Could you check a few things on this drawing? It's one solid part, dimensions in mm from its lowest x, y, z. A direction names the side the tool comes from. Give positions to 0.01 mm unless a question says otherwise; leave off trailing zeros. Order: outer loops, then holes, each group sorted by start corner. A loop starts at its lowest first (then second) coordinate and runs counter-clockwise, first axis right, second up.
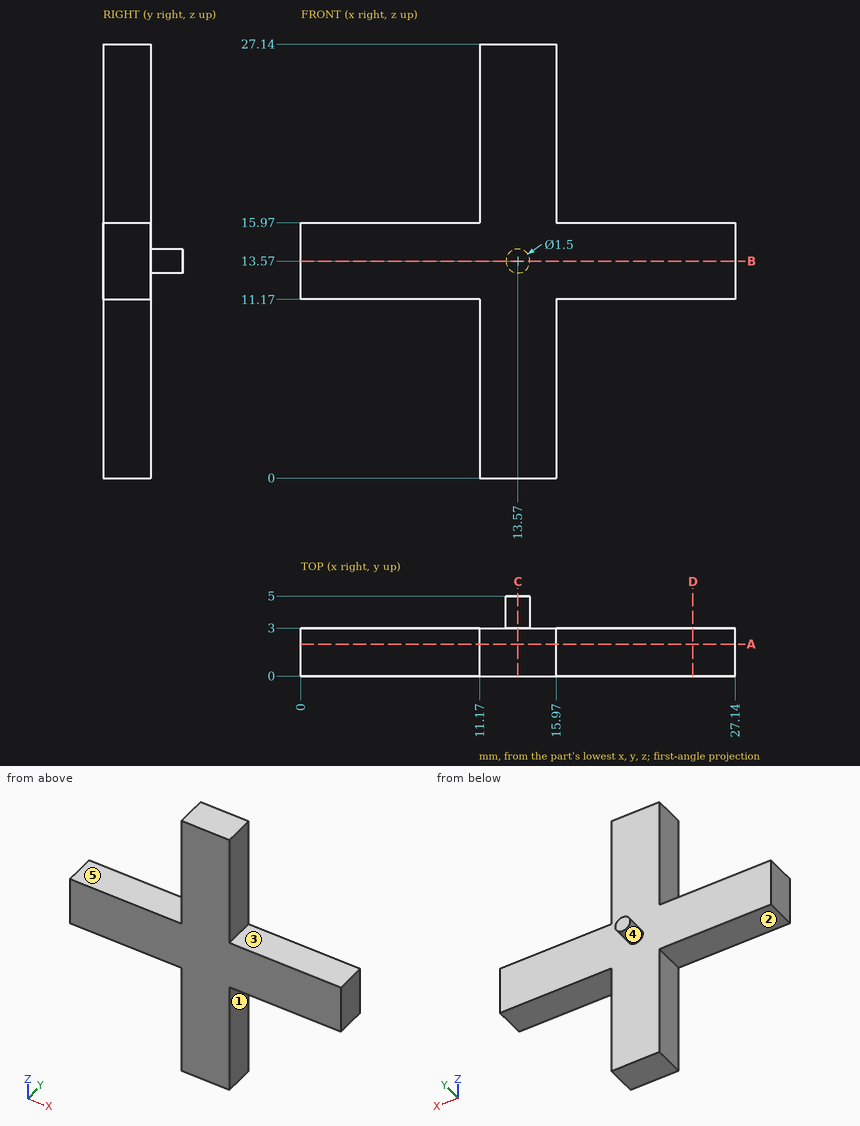
1) Suppose I cut it at A-A (y = 2). Please give me the cut outline in (x, z).
2) Suppose I cut it at D-D (x = 24.5). Please give me the cut outline in (y, z), and give its area (3 significant figures).
3) Suppose I cut it at B-B (z = 13.57). Please give me the cut outline in (x, y), and give its area (3 significant figures).
4) I'm going to push flat-ended pins straight in: pin 1 Ø2.5 at (y, z) = (1, 20.5) entering from +X; pin 2 Ø0.9 at (y, z) = (1, 4) entering from -X; pin 3 Ø1.5 at (x, y) = (6, 1) entering from +Z. Where does each tip first touch, or does it pass through?
5) Which directions (+Z, -Z, +X, -X, +Y, -Y) give clear straight access to the entire face, cutting with the end or side of a thin tool? Please do the marked faces 1, 2, 3, 4 and 5.
6) If I drill on line 1 (Z direction, x = 19.25, y = 1.75); line 2 (Z direction, x = 13.5, y = 4.45), over which ranges is the centre line in solid material (lowest first)?
7) Suppose I cut it at C-C (x = 13.57). Please give me the cut outline in (y, z).
Results:
1. outline: (0, 11.17) - (11.17, 11.17) - (11.17, 0) - (15.97, 0) - (15.97, 11.17) - (27.14, 11.17) - (27.14, 15.97) - (15.97, 15.97) - (15.97, 27.14) - (11.17, 27.14) - (11.17, 15.97) - (0, 15.97) - close
2. outline: (0, 11.17) - (3, 11.17) - (3, 15.97) - (0, 15.97) - close
2. area: 14.4 mm2
3. outline: (0, 0) - (27.14, 0) - (27.14, 3) - (14.32, 3) - (14.32, 5) - (12.82, 5) - (12.82, 3) - (0, 3) - close
3. area: 84.4 mm2
4. pin 1: stops at x = 15.97
4. pin 2: stops at x = 11.17
4. pin 3: stops at z = 15.97
5. face 1: -Z, +X, +Y, -Y
5. face 2: -Z, -X, +Y, -Y
5. face 3: +Z, +X, +Y, -Y
5. face 4: +Y
5. face 5: +Z, -X, +Y, -Y
6. line 1: z = 11.17 to 15.97
6. line 2: z = 12.82 to 14.32
7. outline: (0, 0) - (3, 0) - (3, 12.82) - (5, 12.82) - (5, 14.32) - (3, 14.32) - (3, 27.14) - (0, 27.14) - close
